Can you work these out from the model? Positions are in its coordinate system, mm. A direction names the side the tool comes from. Coordinates: 2 decimals unless noted, no trailing zeros. Order: outer loops, then holes, each group sorted by start corner. A loop starts at its lowest first (then second) coordinate and runs counter-clockwise, first axis right, second up. Notation, with made-up numbers: (25, -14) - (52, -14) arc R28 ccw to (52, 22) - close; hole circle Ø9 at (83, -17). An arc over 180 degrees is marked (long way). Use a Markdown table: item, result. Add a question column.
(1) I want a section at A-A (z = 10). List the corners of the cut face in (x, y) for me.
(2) For pin 1 Ø1.5 at (x, y) = (14.5, 7) entering from +Z; pin 2 Ø2.5 at (x, z) = (7.5, 10) entering from +Y; pin 3 Ø4 at (y, z) = (4.5, 13.5) entering from -X, each with a flat end and sliding along its axis, tell me the tip position at first contact or that it passes through.
(3) On a 3-axis mill with a long thin cutter (end or side, diameter ignored), from which of +Z, -Z, +X, -X, +Y, -Y can I reach the whole of each face in a straight line? I mean faces 1 (the cylindrical face through (13.5, 6.57, 19.01)), 2 (the flat face through (15, 9, 20)), 3 (the cylindrical face through (21.3, 12, 10.9)). Say none if no direction works.
(4) We'd pull the mould along Z, two halves only. Please class faces 4 (the flat face through (15, 0, 10)), 5 (the flat face through (22, 11, 10)), 6 (the flat face through (15, 7, 18)): pulls with the +Z half, pulls with the -Z half, needs draft (parallel to the pull), parting line crosses it, or undercut.
(5) If I drill on L1, parallel to X at y = 11.9, z = 10; L2, parallel to Z at x = 22.5, y = 11.85; L3, parallel to Y at x = 15, z = 18.7, over which ranges is the centre line in solid material (lowest first)? Write a range as [from, to].
(6) I want a section at B-B (x = 7.5). List the corners of the cut face in (y, z) for me, and give its area (3 significant figures).
```python
from build123d import *

# Parameters (mm, degrees)
SKETCH1_W           = 30
SKETCH1_H           = 13
BOSS_EXTRUDE1_DEPTH = 20
SKETCH2_R           = 1.5
CUT_EXTRUDE1_DEPTH  = 2
SKETCH3_R           = 1.5
CUT_EXTRUDE2_DEPTH  = 2


with BuildPart() as part:
    # Sketch1 → Boss-Extrude1 (new body)
    with BuildSketch(Plane.XY):
        with Locations((15, 6.5)):
            Rectangle(SKETCH1_W, SKETCH1_H)
    extrude(amount=BOSS_EXTRUDE1_DEPTH)

    # Sketch2 → Cut-Extrude1 (cut)
    with BuildSketch(Plane.XY.offset(20)):
        with Locations((15, 6.5)):
            Circle(SKETCH2_R)
    extrude(amount=-CUT_EXTRUDE1_DEPTH, mode=Mode.SUBTRACT)

    # Sketch3 → Cut-Extrude2 (cut)
    with BuildSketch(Plane(origin=(0, 13, 0), x_dir=(1, 0, 0), z_dir=(0, 1, 0))):
        with Locations((7.5, -10)):
            Circle(SKETCH3_R)
        with Locations((22.5, -10)):
            Circle(SKETCH3_R)
    extrude(amount=-CUT_EXTRUDE2_DEPTH, mode=Mode.SUBTRACT)


solid = part.part
```
Answers follow:
| question | item | result |
|---|---|---|
| 1 | outline | (0, 0) - (30, 0) - (30, 13) - (24, 13) - (24, 11) - (21, 11) - (21, 13) - (9, 13) - (9, 11) - (6, 11) - (6, 13) - (0, 13) - close |
| 2 | pin 1 | stops at z = 18 |
| 2 | pin 2 | stops at y = 11 |
| 2 | pin 3 | stops at x = 0 |
| 3 | face 1 | +Z |
| 3 | face 2 | +Z, +X, -X, +Y, -Y |
| 3 | face 3 | +Y |
| 4 | face 4 | needs draft |
| 4 | face 5 | undercut |
| 4 | face 6 | pulls with the +Z half |
| 5 | L1 | x = [0, 6], [9, 21], [24, 30] |
| 5 | L2 | z = [0, 8.5], [11.5, 20] |
| 5 | L3 | y = [0, 5], [8, 13] |
| 6 | outline | (0, 0) - (13, 0) - (13, 8.5) - (11, 8.5) - (11, 11.5) - (13, 11.5) - (13, 20) - (0, 20) - close |
| 6 | area | 254 mm² |
